```python
from build123d import *

# Parameters (mm, degrees)
F1_DEPTH    = 2
F3_DEPTH    = 1
F5_DEPTH    = 25
F6_T1_DEPTH = 3.532364341


# Not quite as in the source:
# - a fillet or chamfer that OpenCascade refuses, or shapes differently, is made with other operations: its cross-section is extruded or revolved along the edge and cut away or added


with BuildPart() as f1:
    # F0 (on Top) → F1 (new body)
    with BuildSketch(Plane.XY):
        with BuildLine():
            Line((56.2581913165, 7.0569766727), (11.7505642065, 22.2513897102))
            ThreePointArc((11.7505642065, 22.2513897102), (-21.3224604142, -1.8547742058), (12.5910944331, -24.7633510695))
            Line((12.5910944331, -24.7633510695), (56.5271609891, -7.9877403768))
            ThreePointArc((56.5271609891, -7.9877403768), (59.80596685, -5.6514457625), (61.5316564147, -2.0140241586))
            Line((61.5316564147, -2.0140241586), (53.6735452507, -2.0140241586))
            Line((53.6735452507, -2.0140241586), (53.6735452507, 1.1534155326))
            Line((53.6735452507, 1.1534155326), (61.4978499313, 1.1534155326))
            ThreePointArc((61.4978499313, 1.1534155326), (59.6568196422, 4.7964129612), (56.2581913165, 7.0569766727))
        make_face()
        with BuildLine():
            ThreePointArc((-9.6162715523, -17.7966343508), (-17.1193131366, 2.1791704159), (-3.3569313702, 18.4863852979))
            Line((-3.3569313702, 18.4863852979), (-3.0737131177, 17.6849569346))
            ThreePointArc((-3.0737131177, 17.6849569346), (7.1161082705, 18.5473361415), (16.4279902868, 14.3206339835))
            Line((16.4279902868, 14.3206339835), (16.9633620538, 14.9808438525))
            ThreePointArc((16.9633620538, 14.9808438525), (24.466403638, -4.9949609142), (10.7040218716, -21.3021757961))
            Line((10.7040218716, -21.3021757961), (10.4208036191, -20.5007474329))
            ThreePointArc((10.4208036191, -20.5007474329), (0.2309822309, -21.3631266398), (-9.0808997854, -17.1364244817))
            Line((-9.0808997854, -17.1364244817), (-9.6162715523, -17.7966343508))
        make_face(mode=Mode.SUBTRACT)
    extrude(amount=F1_DEPTH)

    # F2 (on face) → F3 (join)
    with BuildSketch(Plane.XY.offset(2)):
        with BuildLine():
            ThreePointArc((53.6735452507, 1.1654510324), (36.4234102314, 5.106684653), (22.0966452002, 15.4914949248))
            ThreePointArc((22.0966452002, 15.4914949248), (17.3479051946, 19.5208381125), (11.7505642065, 22.2513897102))
            ThreePointArc((11.7505642065, 22.2513897102), (-21.3224604142, -1.8547742058), (12.5910944331, -24.7633510695))
            ThreePointArc((12.5910944331, -24.7633510695), (18.1068462898, -21.8206319867), (22.7200407832, -17.6014435919))
            ThreePointArc((22.7200407832, -17.6014435919), (36.6180007946, -6.6981986771), (53.6735452507, -2.100107176))
            Line((53.6735452507, -2.100107176), (53.6735452507, -2.0140241586))
            Line((53.6735452507, -2.0140241586), (53.6735452507, 1.1534155326))
            Line((53.6735452507, 1.1534155326), (53.6735452507, 1.1654510324))
        make_face()
        with BuildLine():
            ThreePointArc((16.9633620538, 14.9808438525), (22.7211846654, 7.6694079147), (24.7735452507, -1.4078952491))
            ThreePointArc((24.7735452507, -1.4078952491), (20.9007484001, -13.591222859), (10.7040218716, -21.3021757961))
            ThreePointArc((10.7040218716, -21.3021757961), (0.0864795857, -22.2007536364), (-9.6162715523, -17.7966343508))
            ThreePointArc((-9.6162715523, -17.7966343508), (-17.1193131366, 2.1791704159), (-3.3569313702, 18.4863852979))
            ThreePointArc((-3.3569313702, 18.4863852979), (7.2606109157, 19.3849631382), (16.9633620538, 14.9808438525))
        make_face(mode=Mode.SUBTRACT)
    extrude(amount=F3_DEPTH)

    # F4 (on face) → F5 (cut)
    with BuildSketch(Plane(origin=(0, 0, 0), x_dir=(1, 0, 0), z_dir=(0, 0, -1))):
        Polygon((-8.5801632286, 17.98029692), (-8.4723387845, 17.2191802412), (-7.1583543904, 18.1015189737), (-7.951295166, 18.4884736217), align=None)
        Polygon((15.7582396641, -15.4063906521), (15.5428694561, -14.4470129162), (14.0254860744, -15.2497580275), (14.9163370952, -15.9154478461), align=None)
    extrude(amount=-F5_DEPTH, mode=Mode.SUBTRACT)

    # F6: chamfer of 0.3 on 4 edges, made by hand

    # F6_s2 → F6_t1 (cut)
    with BuildSketch(Plane.XY.offset(-0.7661821705)):
        with BuildLine():
            Line((-9.2684752215, -17.3677387978), (-8.8499270506, -17.3209446589))
            ThreePointArc((-8.8499270506, -17.3209446589), (-8.9624343354, -17.2317544465), (-9.0808997854, -17.1364244817))
            Line((-9.0808997854, -17.1364244817), (-9.2684752215, -17.3677387978))
        make_face()
        with BuildLine():
            Line((10.5200333329, -20.7815397421), (10.1413568327, -20.5972129374))
            ThreePointArc((10.1413568327, -20.5972129374), (10.2772447573, -20.5508744537), (10.4208036191, -20.5007474329))
            Line((10.4208036191, -20.5007474329), (10.5200333329, -20.7815397421))
        make_face()
        with BuildLine():
            Line((16.6155657229, 14.5519482995), (16.197017552, 14.5051541606))
            ThreePointArc((16.197017552, 14.5051541606), (16.3095248368, 14.4159639483), (16.4279902868, 14.3206339835))
            Line((16.4279902868, 14.3206339835), (16.6155657229, 14.5519482995))
        make_face()
        with BuildLine():
            Line((-2.7942663313, 17.7814224391), (-3.1729428315, 17.9657492438))
            Line((-3.1729428315, 17.9657492438), (-3.0737131177, 17.6849569346))
            ThreePointArc((-3.0737131177, 17.6849569346), (-2.9301542559, 17.7350839554), (-2.7942663313, 17.7814224391))
        make_face()
    extrude(amount=F6_T1_DEPTH, mode=Mode.SUBTRACT)


solid = f1.part
```
Could you check a few things on this model? Use its own coordinates, in mm. A direction names the side the tool comes from. Give positions to 0.01 mm unless a question says otherwise; leave off trailing zeros. Write each loop counter-clockwise with the first axis right and the second up, starting at its lowest first coordinate (ties: lowest second). Pieces come first, ordered by that corner, then holes. Notation, with made-up numbers: (89, 7.25) - (104, 7.25) arc R35 ccw to (104, 45.25) - close; hole circle Ø10 at (-20, 76.5). An arc over 180 degrees is marked (long way). One line per item, written item: value. Start each with the question number.
Item 1: Imagine slicing it at B-B, the plane x = -16. List the corners of the cut face in (y, z) for me.
Item 2: Imagine slicing it at C-C, the plane y = -12. List the corners of the cut face in (x, z) for me, and give its area (3 significant figures).
Item 3: I'm going to push flat-ended pins straight in: pin 1 (5.5 mm diameter, centred on x = 6.5, y = 16.5, fed in from +Z); pin 2 (11.5 mm diameter, centred on x = 37.5, y = -8, fed in from +Z); pin 3 (1 mm diameter, centred on x = 57, z = 1, fed in from +Y); pin 4 (1 mm diameter, centred on x = 59, z = 1, fed in from -Y). Where does each tip first touch, or does it pass through?
Item 4: Please list where these lines run through material, in increasing order: line 1 (X direction, y = -1, z = 1.2); line 2 (X direction, y = -3.5, z = 1.35); line 3 (Y direction, x = 22.5, z = 2.55). Write a range as from..to.
Item 5: Imagine slicing it at A-A, the plane z = 2.5. List the corners of the cut face in (x, y) for me.
Item 6: Imagine slicing it at D-D, the plane x = 35.5. List the corners of the cut face in (y, z) for me.
Item 7: If we mould it in two halves opening along X, with no side actions, what happens to faces 1 (the face through (0, -22, 2)), 2 (the face through (6, 18.71, 0.99)), 3 (the face through (36.651, 5.004, 2.493)), 4 (the face through (24.3, -6.8, 3))? For each: +X half, -X half, draft (parallel to the pull), parting line (faces both ways), or undercut.
Item 8: Which directions (+Z, -Z, +X, -X, +Y, -Y) give clear straight access to the entire face, cutting with the end or side of a thin tool? Please do faces 5 (the face through (58, 1.153, 1)), 6 (the face through (36.4, -6.81, 2.49)), 7 (the face through (40, 9, 2)), 8 (the face through (7, 19, 2)).
Geometry says:
1. outline: (-16.83, 0) - (-9.03, 0) - (-9.03, 3) - (-16.83, 3) - close; (6.22, 0) - (14.02, 0) - (14.02, 3) - (6.22, 3) - close
2. outline: (-18.97, 0) - (-14.58, 0) - (-14.58, 3) - (-18.97, 3) - close; (21.92, 0) - (46.02, 0) - (46.02, 2) - (28.43, 2) - (28.43, 3) - (21.92, 3) - close
2. area: 67.9 mm^2
3. pin 1: z = 2
3. pin 2: z = 3
3. pin 3: y = 6.97
3. pin 4: y = -6.89
4. line 1: -21.32..-17.42, 24.77..53.67
4. line 2: -21.24..-17.32, 24.67..61.1
4. line 3: -17.86..-10.94, 8.12..15.06
5. outline: (22.1, 15.49) arc R25 ccw (long way) to (22.72, -17.6) arc R44.25 cw to (53.67, -2.1) - (53.67, 1.17) arc R44.25 cw to start; hole circle Ø42.2 at (3.67, -1.41)
6. outline: (-16.02, 0) - (14.14, 0) - (14.14, 2) - (5.54, 2) - (5.54, 3) - (-7.28, 3) - (-7.28, 2) - (-16.02, 2) - close
7. face 1: undercut
7. face 2: undercut
7. face 3: +X half
7. face 4: draft
8. face 5: +Z, -Z, +X
8. face 6: +Z, +X, -Y
8. face 7: +Z, +X, +Y
8. face 8: +Z
